Geometry: final body of the model. Coordinates: model frame, mm. A direction names the side the tool comes from. Give positions to 0.01 mm unless a question says otherwise; leave off trailing zeros. Loops run counter-clockwise (first coordinate to the right, second up) from the corner with the lowest first, then second, coordinate; pieces in that order, holes last. Notation, with made-up numbers: (81.5, -25) -> (130.5, -25) arc R6 cw to (130.5, -14) -> close; hole circle Ø6 at (-3.5, -15). An arc over 180 degrees is marked (long way). One line per question, with ' | ' between items. Start each with the question number.
Item 1: Pin query (flat end, axial travel): P1, Ø5, axis at y = -3.5, z = -9.5, coming from the +X side; P2, Ø1, axis at x = -29, y = -8.5, coming from the +Z side; P3, Ø5, axis at y = -4, z = -38, coming from the +X side. Return the tip coordinate at first contact, or that it passes through.
Item 2: Material intervals for line 1 along X through (y, z) = (-7, -14.5); line 2 along Z through (x, y) = (40, -13); line 3 along X through (y, z) = (-0.75, 10), sorted ascending. Write a range as [from, to].
Item 3: Section B-B on x = 0. Return loops of the section in (y, z).
Item 4: Section A-A on z = 0. Return loops of the section in (x, y).
Item 5: Set-up query: faces 5 (the cylindrical face through (-34.96, -11.02, 40)), 6 (the cylindrical face through (45.676, -2.986, -2.01)). Return all of +Z, -Z, +X, -X, +Y, -Y with unobstructed straight access to the full face (end or side cutting, diameter ignored); none if empty.
Item 6: Section D-D on z = 50.5. Return loops of the section in (x, y), then the cut area to 3 significant figures.
Item 7: Mould query, pull axis Z, two halves, no side actions, for faces 1 (the cylindrical face through (-58.677, -11.017, 2.582)), 2 (the cylindrical face through (-36.818, -11.017, -41.076)), 3 (the flat face through (-17, -4.75, 43)), 4 (the cylindrical face through (31.24, -8.61, -23.96)). Classes: released by +Z, released by -Z, zero draft, split by the parting line, or undercut.
Item 8: Section C-C on y = -3.25. Return loops of the section in (x, z).
from build123d import *

# Parameters (mm, degrees)
F0_R     = 58.7341750738
F1_DEPTH = 17.4625
F2_W     = 17.6311007185
F2_H     = 8.097752736
F4_SIZE  = 1.27
F6_D     = 7.1374
F7_D     = 78.74


with BuildPart() as f1:
    # F0 (on Front) → F1 (new body)
    with BuildSketch(Plane.XZ):
        Circle(F0_R)
    extrude(amount=F1_DEPTH)

    # F2 (on Top) → F3 (revolve, cut)
    with BuildSketch(Plane.XY):
        with Locations((-54.5355503593, -0.700923632)):
            Rectangle(F2_W, F2_H)
    revolve(axis=Axis((0, -1.8075983971, 0), (0, -1, 0)), mode=Mode.SUBTRACT)

    # F4
    f4_edges = [f1.edges().sort_by_distance(p)[0] for p in [
        (45.72, 0, 0),
    ]]
    chamfer(f4_edges, length=F4_SIZE)

    # F6 (through all)
    with Locations(Plane.XZ.offset(17.4625)):
        with Locations((-37.592, 37.592), (37.592, 37.592), (37.592, -37.592), (-37.592, -37.592)):
            Hole(F6_D / 2)

    # F7 (through all)
    with Locations(Plane.XZ.offset(17.4625)):
        with Locations((0, 0)):
            Hole(F7_D / 2)


solid = f1.part
Result sheet:
1) P1: stops at x = 58.27 | P2: stops at z = 51.36 | P3: stops at x = 46.7
2) line 1: x = [-56.92, -36.6], [36.6, 56.92] | line 2: z = [-43.01, -40.23], [-34.96, 34.96], [40.23, 43.01] | line 3: x = [-44.08, -38.08], [38.08, 44.08]
3) outline: (-17.46, -58.73) -> (-4.75, -58.73) -> (-4.75, -45.72) -> (-1.27, -45.72) -> (0, -44.45) -> (0, -39.37) -> (-17.46, -39.37) -> close; (-17.46, 39.37) -> (0, 39.37) -> (0, 44.45) -> (-1.27, 45.72) -> (-4.75, 45.72) -> (-4.75, 58.73) -> (-17.46, 58.73) -> close
4) outline: (-58.73, -17.46) -> (-39.37, -17.46) -> (-39.37, 0) -> (-44.45, 0) -> (-45.72, -1.27) -> (-45.72, -4.75) -> (-58.73, -4.75) -> close; (39.37, -17.46) -> (58.73, -17.46) -> (58.73, -4.75) -> (45.72, -4.75) -> (45.72, -1.27) -> (44.45, 0) -> (39.37, 0) -> close
5) face 5: +Y, -Y | face 6: +Y
6) outline: (-29.99, -17.46) -> (29.99, -17.46) -> (29.99, -4.75) -> (-29.99, -4.75) -> close | area: 763 mm²
7) face 1: split by the parting line | face 2: undercut | face 3: zero draft | face 4: undercut
8) outline: circle Ø91.44 at (0, 0); hole circle Ø78.74 at (0, 0)
